```python
from build123d import *

# Parameters (mm, degrees)
BOSS_EXTRUDE1_DEPTH = 26
SHELL1_T            = -2
CUT_EXTRUDE1_REACH  = 90.591
SKETCH2_W           = 13.02701198
SKETCH2_H           = 22
FILLET1_R           = 1


with BuildPart() as part:
    # Sketch1 → Boss-Extrude1 (new body)
    with BuildSketch(Plane.XY):
        Polygon((0, 0), (-17.764107246, 0), (32.990484886, 80), (32.990484886, 52), align=None)
    extrude(amount=BOSS_EXTRUDE1_DEPTH)

    # Shell1
    shell1_openings = [part.faces().sort_by_distance(p)[0] for p in [
        (32.990484886, 66, 13),
    ]]
    offset(amount=SHELL1_T, openings=shell1_openings, kind=Kind.INTERSECTION)

    # Sketch2 → Cut-Extrude1 (cut, up to next)
    with BuildSketch(Plane(origin=(0, 2, 0), x_dir=(1, 0, 0), z_dir=(0, 1, 0)), mode=Mode.PRIVATE) as cut_extrude1_sk1:
        with Locations((-7.61318882, -13)):
            Rectangle(SKETCH2_W, SKETCH2_H)
    cut_extrude1_tool1 = extrude(cut_extrude1_sk1.sketch, amount=-CUT_EXTRUDE1_REACH, mode=Mode.PRIVATE) & part.part
    add(cut_extrude1_tool1.solids().sort_by_distance((-7.613189, 2, 13))[0], mode=Mode.SUBTRACT)

    # Fillet1
    fillet1_edges = [part.edges().sort_by_distance(p)[0] for p in [
        (7.61318882, 40, 26),
        (16.495242443, 26, 26),
        (7.61318882, 40, 0),
        (16.495242443, 26, 0),
    ]]
    fillet(fillet1_edges, radius=FILLET1_R)


solid = part.part
```
Here's how the part is built. I have some questions about the finished solid (model axes, mm). A direction names the side the tool comes from. Give positions to 0.01 mm unless a question says otherwise; leave off trailing zeros. Order: outer loops, then holes, each group sorted by start corner. A loop starts at its lowest first (then second) coordinate and runs counter-clockwise, first axis right, second up. Notation, with made-up numbers: (4.5, 20.5) - (8.5, 20.5) arc R8 cw to (8.5, 28.5) - close; hole circle Ø4 at (-40, 2.5). An arc over 180 degrees is marked (long way). Answer as a JSON object with one key per item and string values. Group by question number.
Item 1: If we mould it in two halves opening along Y, with no side actions, what happens to faces 1 (the flat face through (7.26, 39.44, 12.83)), 2 (the flat face through (16.18, 29.24, 12.85)), 3 (the cylindrical face through (16.267, 26.173, 0.301))? For each: pulls with the +Y half, pulls with the -Y half, needs draft (parallel to the pull), parting line crosses it, or undercut.
Item 2: Which directions (+Z, -Z, +X, -X, +Y, -Y) give clear straight access to the entire face, cutting with the end or side of a thin tool? Please do faces 4 (the flat face through (11, 33, 2)), 5 (the flat face through (12, 33, 0)), 6 (the flat face through (-14.127, 1, 13)).
Item 3: Please list where these lines run through material, in increasing order: probe 1 along Z at (x, y) = (23, 46); probe 2 along Y at (x, z) = (6, 7.5); probe 3 along X at (y, z) = (30.5, 14.75).
Item 4: If we section it at A-A on z = 9.25: Please give me the cut outline in (x, y), and give its area (3 significant figures).
Item 5: For P1, Ø4, axis at y = 10, z = 17, coming from the -X side; P2, Ø1, axis at y = 1.5, z = 17.5, coming from the +X side; P3, Ø8, axis at y = 13, z = 21.5, coming from the +X side, each with a flat end and sliding along its axis, tell me the tip position at first contact or that it passes through.
Result set:
{
 "1": {"face 1": "pulls with the +Y half", "face 2": "undercut", "face 3": "pulls with the -Y half"},
 "2": {"face 4": "none", "face 5": "-Z, +X, -X, +Y, -Y", "face 6": "-Y"},
 "3": {"probe 1": "0 to 2, 24 to 26", "probe 2": "9.46 to 13.19, 33.72 to 37.46", "probe 3": "1.59 to 3.95, 16.98 to 19.35"},
 "4": {"outline": "(-17.76, 0) - (-14.13, 0) - (-14.13, 2) - (32.99, 76.27) - (32.99, 80) - close; (-1.1, 0) - (0, 0) - (32.99, 52) - (32.99, 55.73) - (-1.1, 2) - close", "area": "313 mm²"},
 "5": {"P1": "x = -12.69", "P2": "x = 1.27", "P3": "x = 10.79"}
}
